Work out the finished part from the listing and answer in its coordinate system (mm). A direction names the side the tool comes from. Coordinates: 2 decimals unless noted, no trailing zeros. Order: outer loops, then holes, each group sorted by start corner. A loop starts at its lowest first (then second) coordinate and runs counter-clockwise, first axis right, second up. Notation, with made-up numbers: (-20.75, -16) - (0.25, -16) arc R22 ccw to (0.25, 3) - close; hole circle Ø6 at (6, -6). An arc over 180 degrees is marked (long way). Answer as a JSON object with one key per item and string values. Group by question number.
1) Section A-A (x = 0) is taken. Give the vertices of the cut face in (y, z) (1 decimal).
2) Section D-D (x = -2.25) is taken. Give the vertices of the cut face in (y, z) (3 decimals).
3) Section C-C (z = -13.75) is taken. Give the vertices of the cut face in (x, y), plus the area to 3 significant figures.
4) Find the intervals of material crossed by line 1 along Z through (x, y) = (2, 4.25) (3 decimals); line 2 along Y through (x, z) = (0.25, -13.5); line 3 along X through (y, z) = (-0.25, -13), in increasing order.
5) Each of these flat-tipped pins is pushed along its axis until it touches: P1, Ø1.5, axis at x = -3.5, y = 1.5, coming from the -Z side; P2, Ø1, axis at x = 3, z = -4, coming from the +Y side; P3, Ø1.5, axis at x = 0.5, z = -8.5, coming from the -Y side. Where does it stop, or does it pass through?
6) Section B-B (y = 0) is taken. Give the vertices of the cut face in (x, z) (3 decimals).
7) A tool of negligible diameter and unlimited length cuts with its end or side. For faces 1 (the face through (1.524, 0, -10)), 2 (the face through (0, 0.889, -1)), 3 (the face through (0, 1.968, -10)), 4 (the face through (-1.524, 0, -10)), 5 (the face through (0, -1.968, -10)), from which of +Z, -Z, +X, -X, +Y, -Y can it reach the whole face along a straight path? Write none if from no direction.
8) The mould has two halves that part along Z. Classify faces 6 (the face through (-2, -4, -3.175)), 7 (the face through (0, -2, 0)), 8 (the face through (0, 0, -14.859)), 9 (the face through (-0.853, 3.843, -3.676)): released by +Z, released by -Z, zero draft, split by the parting line, or undercut.
from build123d import *

# Parameters (mm, degrees)
F0_R     = 4.826
F1_DEPTH = 3.175
F2_W     = 11.9897948747
F2_H     = 1.778
F3_DEPTH = 2.286
F4_R     = 3.937
F5_DEPTH = 1.016
F6_R     = 4.826
F7_DEPTH = 0.762
F8_W     = 3.048
F8_H     = 3.937
F9_DEPTH = 9.906


# Not quite as in the source:
# - the program builds the solid bodies; features that only make, move or delete a surface that nothing else refers to are left out


with BuildPart() as f1:
    # F0 (on Top) → F1 (new body)
    with BuildSketch(Plane.XY):
        Circle(F0_R)
    extrude(amount=-F1_DEPTH)

    # F2 (on face) → F3 (cut)
    with BuildSketch(Plane.XY):
        Rectangle(F2_W, F2_H)
    extrude(amount=-F3_DEPTH, mode=Mode.SUBTRACT)

    # F4 (on face) → F5 (join)
    with BuildSketch(Plane(origin=(0, 0, -3.175), x_dir=(1, 0, 0), z_dir=(0, 0, -1))):
        Circle(F4_R)
    extrude(amount=F5_DEPTH)

    # F6 (on face) → F7 (join)
    with BuildSketch(Plane(origin=(0, 0, -4.191), x_dir=(1, 0, 0), z_dir=(0, 0, -1))):
        Circle(F6_R)
    extrude(amount=F7_DEPTH)

    # F8 (on face) → F9 (join)
    with BuildSketch(Plane(origin=(0, 0, -4.953), x_dir=(1, 0, 0), z_dir=(0, 0, -1))):
        Rectangle(F8_W, F8_H)
    extrude(amount=F9_DEPTH)


solid = f1.part
Report:
{
 "1": {"outline": "(-4.8, -5) - (-2, -5) - (-2, -14.9) - (2, -14.9) - (2, -5) - (4.8, -5) - (4.8, -4.2) - (3.9, -4.2) - (3.9, -3.2) - (4.8, -3.2) - (4.8, 0) - (0.9, 0) - (0.9, -2.3) - (-0.9, -2.3) - (-0.9, 0) - (-4.8, 0) - (-4.8, -3.2) - (-3.9, -3.2) - (-3.9, -4.2) - (-4.8, -4.2) - close"},
 "2": {"outline": "(-4.269, -4.953) - (4.269, -4.953) - (4.269, -4.191) - (3.231, -4.191) - (3.231, -3.175) - (4.269, -3.175) - (4.269, 0) - (0.889, 0) - (0.889, -2.286) - (-0.889, -2.286) - (-0.889, 0) - (-4.269, 0) - (-4.269, -3.175) - (-3.231, -3.175) - (-3.231, -4.191) - (-4.269, -4.191) - close"},
 "3": {"outline": "(-1.52, -1.97) - (1.52, -1.97) - (1.52, 1.97) - (-1.52, 1.97) - close", "area": "12.0 mm²"},
 "4": {"line 1": "z = -4.953 to -4.191, -3.175 to 0", "line 2": "y = -1.97 to 1.97", "line 3": "x = -1.52 to 1.52"},
 "5": {"P1": "stops at z = -4.95", "P2": "stops at y = 4.1", "P3": "stops at y = -1.97"},
 "6": {"outline": "(-4.826, -4.953) - (-1.524, -4.953) - (-1.524, -14.859) - (1.524, -14.859) - (1.524, -4.953) - (4.826, -4.953) - (4.826, -4.191) - (3.937, -4.191) - (3.937, -3.175) - (4.826, -3.175) - (4.826, -2.286) - (-4.826, -2.286) - (-4.826, -3.175) - (-3.937, -3.175) - (-3.937, -4.191) - (-4.826, -4.191) - close"},
 "7": {"face 1": "-Z, +X, +Y, -Y", "face 2": "+Z, +X, -X", "face 3": "-Z, +X, -X, +Y", "face 4": "-Z, -X, +Y, -Y", "face 5": "-Z, +X, -X, -Y"},
 "8": {"face 6": "undercut", "face 7": "released by +Z", "face 8": "released by -Z", "face 9": "undercut"}
}
